The drawing under review shows one solid part. Ordinate dimensions are in mm from its lowest x, y, z. Round coordinates to 2 decimals unless told otherwise and drop trailing zeros. Order: outer loops, then holes, each group sorted by start corner. A loop starts at its lowest first (then second) coordinate and runs counter-clockwise, first axis right, second up.
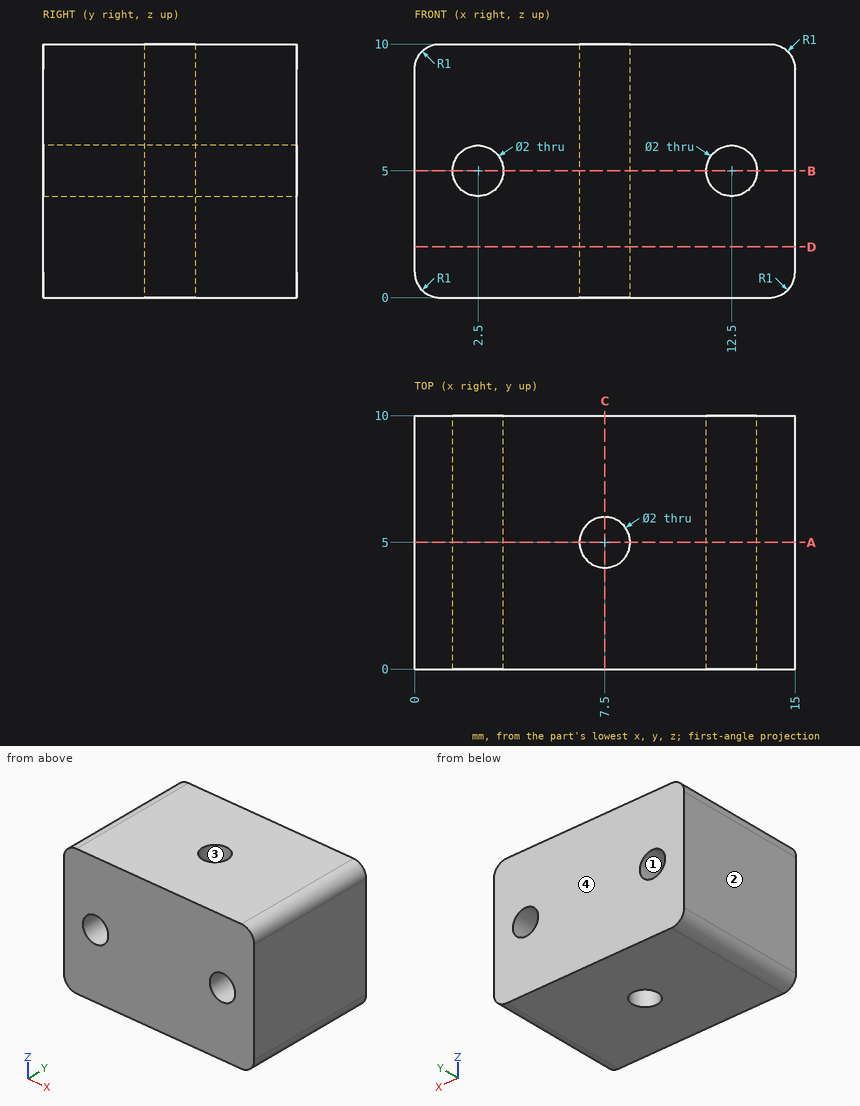
(1) We need section C-C (x = 7.5). Give the boundary of the cut face in (y, z).
(2) We need section A-A (y = 5). Give the boundary of the cut face in (x, z).
(3) We need section B-B (z = 5). Give the boundary of the cut face in (x, y), and give its area (3 significant figures).
(4) Clearance check with a flat-ended pin moving along its axis: P1, Ø1.8, axis at x = 2.5, z = 5, coming from the +Y side. State where the tip first meets the part, or that it passes through.
(5) We need section D-D (z = 2). Give the boundary of the cut face in (x, y).
(6) To check wall thickness, follow L1, parallel to X at y = 2, z = 5; L2, parallel to Y at x = 7.5, z = 3; L3, parallel to X at y = 5.25, z = 4.75. State the ranges of each line that lie inside material, in increasing order.
(7) The part is to be moulded in two halves that separate along X. For the marked faces 1, 2, 3 and 4, say which applies: pulls with the +X half, pulls with the -X half, needs draft (parallel to the pull), parting line crosses it, or undercut.
Verdict:
1. outline: (0, 0) - (4, 0) - (4, 10) - (0, 10) - close; (6, 0) - (10, 0) - (10, 10) - (6, 10) - close
2. outline: (0, 1) arc R1 ccw to (1, 0) - (6.5, 0) - (6.5, 10) - (1, 10) arc R1 ccw to (0, 9) - close; (8.5, 0) - (14, 0) arc R1 ccw to (15, 1) - (15, 9) arc R1 ccw to (14, 10) - (8.5, 10) - close; hole circle Ø2 at (2.5, 5); hole circle Ø2 at (12.5, 5)
3. outline: (0, 0) - (1.5, 0) - (1.5, 10) - (0, 10) - close; (3.5, 0) - (11.5, 0) - (11.5, 10) - (3.5, 10) - close; (13.5, 0) - (15, 0) - (15, 10) - (13.5, 10) - close; hole circle Ø2 at (7.5, 5)
3. area: 107 mm2
4. P1: passes through
5. outline: (0, 0) - (15, 0) - (15, 10) - (0, 10) - close; hole circle Ø2 at (7.5, 5)
6. L1: x = 0 to 1.5, 3.5 to 11.5, 13.5 to 15
6. L2: y = 0 to 4, 6 to 10
6. L3: x = 0 to 1.53, 3.47 to 6.53, 8.47 to 11.53, 13.47 to 15
7. face 1: undercut
7. face 2: pulls with the -X half
7. face 3: undercut
7. face 4: needs draft
